Autodesk Inventor part; units mm, degrees
ref_plane "YZ Plane" through (0, 0, 0) normal (1, 0, 0) x (0, 1, 0)
ref_plane "XZ Plane" through (0, 0, 0) normal (0, 1, 0) x (-1, 0, 0)
ref_plane "XY Plane" through (0, 0, 0) normal (0, 0, 1) x (1, 0, 0)
sketch "スケッチ1" plane through (0, 0, 0) normal (0, 0, 1) x (1, 0, 0)
  circle A0 centre (0, 0) radius 7
  dimension "d0" = 14
extrude "押し出し1" add sketch "スケッチ1" along normal blind 4
sketch "スケッチ2" plane through (0, 0, 0) normal (0, 0, -1) x (-1, 0, 0)
  circle A0 centre (0, 0) radius 7.5
  dimension "d3" = 15
extrude "押し出し2" add sketch "スケッチ2" along normal blind 1
sketch "スケッチ3" plane through (0, 0, 4) normal (0, 0, 1) x (1, 0, 0)
  point P0 (0, 0)
  point P1 (0, 0)
hole "穴1" at (0, 0, 4) direction (0, 0, -1) diameter 5 depth 5 tip angle 118
properties part number "玉軸受1 F605ZZ"
The listing builds one solid part. Answer for the finished solid, in the listing's coordinates (mm). A direction names the side the tool comes from. Coordinates: 2 decimals unless noted, no trailing zeros. Write each loop counter-clockwise with the first axis right and the second up, starting at its lowest first coordinate (ties: lowest second). Pieces come first, ordered by that corner, then holes. Notation, with made-up numbers: (1.5, 88) - (17.5, 88) arc R9 ccw to (17.5, 96) - close; hole circle Ø5 at (-5, 80.25). An arc over 180 degrees is marked (long way). Return JSON: item names as keys, results as strings. Group by question number.
Q1. The part is cut by section A-A on y = 0. Write down the section's boundary in (x, z), and give its area (3 significant figures).
Q2. The part is cut by section D-D on z = 3.3. Write down the section's boundary in (x, y), and give its area (3 significant figures).
Q3. A flat-ended cylindrical pin translates along its axis: pin 1 Ø3 at (x, z) = (-4, 1) entering from -Y. Find the tip coordinate at first contact, or state that the pin passes through.
Q4. The part is cut by section C-C on y = 3.25. Write down the section's boundary in (x, z).
Q5. Which of the six approach directions +Z, -Z, +X, -X, +Y, -Y give full straight-line access (tool end or side, diameter ignored) to faces 1 (the flat face through (2, 2, -1)), 2 (the flat face through (-7, 2, 0))?
Q6. Find the intervals of material crossed by line 1 along Y through (x, z) = (0, 2.1); line 2 along Y through (x, z) = (0, -0.5); line 3 along X through (y, z) = (1.5, 3.55), in increasing order. Write a range as [from, to].
Q7. For a pull along Y with two mould halves and no side action, classify faces 3 (the flat face through (0, -3, 4)), 4 (the cylindrical face through (6.466, 2.681, 1.972)), 5 (the cylindrical face through (2.44, 0.54, 1.46)) as +Y half, -Y half, draft (parallel to the pull), parting line (faces both ways), or undercut.
Evaluation:
{
 "1": {"outline": "(-7.5, -1) - (-2.5, -1) - (-2.5, 4) - (-7, 4) - (-7, 0) - (-7.5, 0) - close; (2.5, -1) - (7.5, -1) - (7.5, 0) - (7, 0) - (7, 4) - (2.5, 4) - close", "area": "46.0 mm2"},
 "2": {"outline": "circle Ø14 at (0, 0); hole circle Ø5 at (0, 0)", "area": "134 mm2"},
 "3": {"pin 1": "stops at y = -6.92"},
 "4": {"outline": "(-6.76, -1) - (6.76, -1) - (6.76, 0) - (6.2, 0) - (6.2, 4) - (-6.2, 4) - (-6.2, 0) - (-6.76, 0) - close"},
 "5": {"face 1": "-Z, +X, -X, +Y, -Y", "face 2": "+Z"},
 "6": {"line 1": "y = [-7, -2.5], [2.5, 7]", "line 2": "y = [-7.5, -2.5], [2.5, 7.5]", "line 3": "x = [-6.84, -2], [2, 6.84]"},
 "7": {"face 3": "draft", "face 4": "parting line", "face 5": "undercut"}
}
